Check sheet for the modelled part. Datum: model origin and axes. Units: mm. Face numbers are marked on the shaded views. A direction names the side the tool comes from. Round coordinates to 2 decimals unless told otherwise and drop trailing zeros. Order: outer loops, then holes, each group sorted by start corner. A loop starts at its lowest first (then second) coordinate and runs counter-clockwise, first axis right, second up.
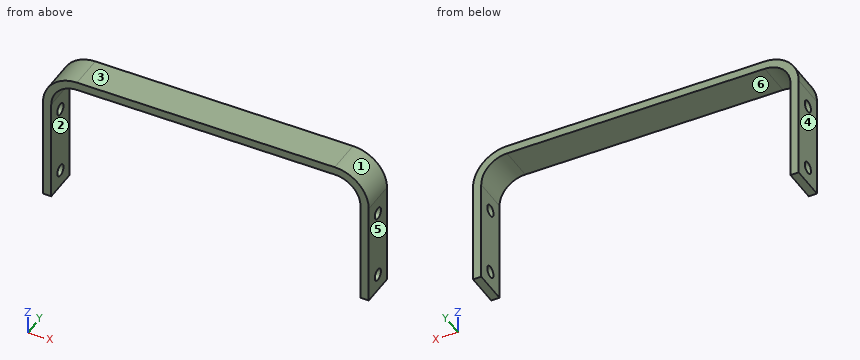
Autodesk Inventor part; units mm, degrees
ref_plane "YZ Plane" through (0, 0, 0) normal (1, 0, 0) x (0, 1, 0)
ref_plane "XZ Plane" through (0, 0, 0) normal (0, 1, 0) x (-1, 0, 0)
ref_plane "XY Plane" through (0, 0, 0) normal (0, 0, 1) x (1, 0, 0)
sketch "Sketch1" plane through (0, 0, 0) normal (0, 0, 1) x (1, 0, 0)
  line L0 (0, 0) -> (-120.396, 0)
  line L1 (-120.396, 0) -> (-120.396, 12.7)
  line L2 (-120.396, 12.7) -> (0, 12.7)
  line L3 (0, 12.7) -> (0, 0)
  dimension "d0" = 120.396
  dimension "d1" = 12.7
extrude "Plate1" add sketch "Sketch1" along normal blind 3.048
sketch "Sketch2" plane through (-3.048, 0, 3.048) normal (1, 0, 0) x (0, 1, 0)
  line L0 (12.7, 0) -> (0, 0)
  line L1 (0, 0) -> (0, -50.673)
  line L2 (0, -50.673) -> (12.7, -50.673)
  line L3 (12.7, -50.673) -> (12.7, 0)
edge flange "Flange1" height 47.625 angle 90 thickness 3.048 bend radius 9.525 thickness toward (1, 0, 0) relief tear relief width 3.048 relief depth 1.524 edges at (0, 6.35, 0) wall of the first edge with corners at (-3.048, 12.7, 3.048) (-3.048, 0, 3.048) (-3.048, 0, -47.625) (-3.048, 12.7, -47.625)
bend "Bend1"
corner "Corner1"
sketch "Sketch3" plane through (-117.348, 12.7, 3.048) normal (-1, 0, 0) x (0, -1, 0)
  line L0 (12.7, 0) -> (0, 0)
  line L1 (0, 0) -> (0, -50.673)
  line L2 (0, -50.673) -> (12.7, -50.673)
  line L3 (12.7, -50.673) -> (12.7, 0)
edge flange "Flange2" height 47.625 angle 90 thickness 3.048 bend radius 9.525 thickness toward (-1, 0, 0) relief tear relief width 3.048 relief depth 1.524 edges at (-120.396, 6.35, 0) wall of the first edge with corners at (-117.348, 0, 3.048) (-117.348, 12.7, 3.048) (-117.348, 12.7, -47.625) (-117.348, 0, -47.625)
bend "Bend2"
corner "Corner2"
sketch "Sketch4" plane through (0, 0, -47.625) normal (1, 0, 0) x (0, 0, -1)
  line L0 (0, 0) -> (-38.1, 0)
  line L1 (0, 12.7) -> (0, 0)
  line L2 (-38.1, 12.7) -> (0, 12.7)
  line L3 (0, 6.35) -> (-6.35, 6.35)
  line L4 (-6.35, 6.35) -> (-31.75, 6.35)
  circle A0 centre (-31.75, 6.35) radius 2.1463
  circle A1 centre (-6.35, 6.35) radius 2.1463
  point P0 (-47.625, 0)
  dimension "d23" = 6.35
  dimension "d24" = 25.4
  dimension "d25" = 4.2926
  dimension "d26" = 4.2926
extrude "Cut1" cut sketch "Sketch4" against normal blind 3.048
sketch "Sketch5" plane through (-120.396, 0, -47.625) normal (-1, 0, 0) x (0, 0, 1)
  line L0 (0, 0) -> (0, 12.7)
  line L1 (38.1, 0) -> (0, 0)
  line L2 (0, 6.35) -> (6.35, 6.35)
  line L3 (6.35, 6.35) -> (31.75, 6.35)
  circle A0 centre (6.35, 6.35) radius 2.1463
  circle A1 centre (31.75, 6.35) radius 2.1463
  point P0 (47.625, 0)
  dimension "d29" = 6.35
  dimension "d30" = 25.4
  dimension "d31" = 4.2926
  dimension "d32" = 4.2926
extrude "Cut2" cut sketch "Sketch5" against normal blind 3.048
equation "\"d27\" = Thickness"
equation "\"d33\" = Thickness"
equation "\"d3\" = BendReliefWidth"
equation "\"d4\" = BendReliefDepth"
equation "\"d5\" = MinimumRemnant"
equation "\"d6\" = BendRadius"
equation "\"d10\" = CornerReliefSize"
equation "\"d11\" = GapSize"
equation "\"d12\" = JacobiRadiusSize"
equation "\"d13\" = BendReliefWidth"
equation "\"d14\" = BendReliefDepth"
equation "\"d15\" = MinimumRemnant"
equation "\"d16\" = BendRadius"
equation "\"d20\" = CornerReliefSize"
equation "\"d21\" = GapSize"
equation "\"d22\" = JacobiRadiusSize"
equation "\"BendRadius\" = Thickness"
equation "\"BendReliefWidth\" = Thickness"
equation "\"BendReliefDepth\" = 0.5 * Thickness"
equation "\"CornerReliefSize\" = 4 * Thickness"
equation "\"MinimumRemnant\" = 2 * Thickness"
equation "\"TransitionRadius\" = BendRadius"
equation "\"JacobiRadiusSize\" = BendRadius"
equation "\"GapSize\" = Thickness"
equation "\"d2\" = BendRadius"
properties part number "Generic brace"
Item 1: Sectioned sample at A-A (y = 6.35). Record the cut outline in (x, z) (3 decimals).
Answer:
outline: (-120.396, -47.625) - (-117.348, -47.625) - (-117.348, -43.421) - (-120.396, -43.421) - close; (-120.396, -39.129) - (-117.348, -39.129) - (-117.348, -18.021) - (-120.396, -18.021) - close; (-120.396, -13.729) - (-117.348, -13.729) - (-117.348, -9.525) arc R9.525 cw to (-107.823, 0) - (-12.573, 0) arc R9.525 cw to (-3.048, -9.525) - (-3.048, -13.729) - (0, -13.729) - (0, -9.525) arc R12.573 ccw to (-12.573, 3.048) - (-107.823, 3.048) arc R12.573 ccw to (-120.396, -9.525) - close; (-3.048, -47.625) - (0, -47.625) - (0, -43.421) - (-3.048, -43.421) - close; (-3.048, -39.129) - (0, -39.129) - (0, -18.021) - (-3.048, -18.021) - close
Item 2: Sectioned sample at C-C (z = -7.5). Record the cut outline in (x, y), and give its area (3 significant figures).
Answer:
outline: (-120.23, 0) - (-117.13, 0) - (-117.13, 12.7) - (-120.23, 12.7) - close; (-3.27, 0) - (-0.16, 0) - (-0.16, 12.7) - (-3.27, 12.7) - close
area: 78.8 mm2
Item 3: Sectioned sample at D-D (x = -50). Record the cut outline in (y, z).
Answer:
outline: (0, 0) - (12.7, 0) - (12.7, 3.05) - (0, 3.05) - close
Item 4: Sectioned sample at B-B (z = -22). Record the cut outline in (x, y), and give its area (3 significant figures).
Answer:
outline: (-120.4, 0) - (-117.35, 0) - (-117.35, 12.7) - (-120.4, 12.7) - close; (-3.05, 0) - (0, 0) - (0, 12.7) - (-3.05, 12.7) - close
area: 77.4 mm2
Item 5: Go/stop test with a flat-tipped pin: P1, Ø4, axis at x = -23, y = 10.5, coming from the -Z side. Record where the tip stops, or that it passes through.
Answer:
P1: stops at z = 0
Item 6: Scan lines: line 1 along X through (y, z) = (2.5, -37); line 2 along Z through (x, y) = (-118.6, 6.35) (3 decimals); line 3 along Z through (x, y) = (-37, 9.25). Record each from-to range of solid material in increasing order.
Answer:
line 1: x = -120.4 to -117.35, -3.05 to 0
line 2: z = -47.625 to -43.421, -39.129 to -18.021, -13.729 to -3.049
line 3: z = 0 to 3.05
Item 7: Access from +Z, -Z, +X, -X, +Y, -Y to the whole of each face (thin tool, end or side, straight path). Record for the marked faces 1 and 2.
Answer:
face 1: +Z, +X, +Y, -Y
face 2: -Z, +Y, -Y
Item 8: Release check for a two-part mould opening along X. For the marked faces 3, 4, 5 and 6 record: released by +X, released by -X, zero draft, split by the parting line, or undercut.
Answer:
face 3: zero draft
face 4: released by -X
face 5: released by +X
face 6: undercut
